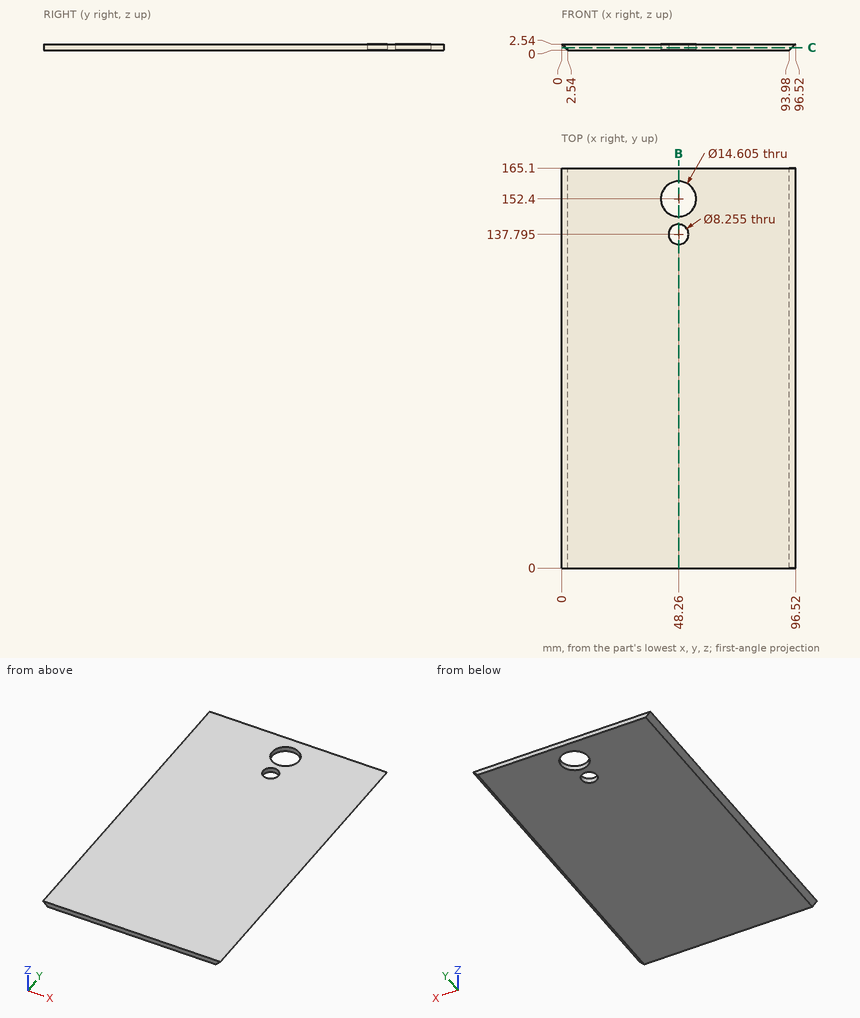
Study the drawing (mm; zero at the part's minimum x, y, z) and answer. Give positions to 0.01 mm unless a question says otherwise; leave off trailing zeros. Write each loop counter-clockwise with the first axis right and the second up, starting at its lowest first coordinate (ties: lowest second). Pieces come first, ordered by that corner, then holes. Notation, with made-up numbers: (3, 10.5) -> (8, 10.5) arc R24 cw to (8, 48.5) -> close; hole circle Ø6 at (-29, 61). An arc over 180 degrees is marked (long way). Answer as a JSON object with one key per item and string values. Group by question number.
1) Consider L1, parallel to Y at x = 48.26, z = 1.4; L2, parallel to X at y = 155.5, z = 0.95; L3, parallel to X at y = 12, z = 1.05. Determine where each line is inside the solid, lowest interval first. Write a range as from..to.
2) Find section B-B (x = 48.26). Write down the section's boundary in (y, z), and give its area (3 significant figures).
3) Find section C-C (z = 1). Write down the section's boundary in (x, y) (1 decimal).
4) Each of these flat-tipped pins is pushed along its axis until it touches: P1, Ø6.5, axis at x = 48.26, y = 137.795, coming from the -Z side; P2, Ø1, axis at y = 64.5, z = 0.5, coming from the -X side. Where does it stop, or does it pass through?
Values follow:
{
 "1": {"L1": "y = 0..133.67, 141.92..145.1, 159.7..165.1", "L2": "x = 1.59..41.65, 54.87..94.93", "L3": "x = 1.49..95.03"},
 "2": {"outline": "(0, 0) -> (133.67, 0) -> (133.67, 2.54) -> (0, 2.54) -> close; (141.92, 0) -> (145.1, 0) -> (145.1, 2.54) -> (141.92, 2.54) -> close; (159.7, 0) -> (165.1, 0) -> (165.1, 2.54) -> (159.7, 2.54) -> close", "area": "361 mm2"},
 "3": {"outline": "(1.5, 0) -> (95, 0) -> (95, 165.1) -> (1.5, 165.1) -> close; hole circle Ø14.6 at (48.3, 152.4); hole circle Ø8.3 at (48.3, 137.8)"},
 "4": {"P1": "passes through", "P2": "stops at x = 1.54"}
}
